The listing builds one solid part. Answer for the finished solid, in the listing's coordinates (mm). Coordinates: 2 decimals unless noted, no trailing zeros. Write each loop counter-clockwise with the first axis right and the second up, starting at its lowest first coordinate (ties: lowest second). Pieces come first, ordered by that corner, then holes. Notation, with made-up numbers: M 25,24 L 55,24 A8 ccw 55,36 Z; hole C -29.75,88 d8. An arc over 180 degrees is marked long. Write item = value, one per line. Start each with the question number.
```python
from build123d import *

# Parameters (mm, degrees)
SKETCH_1_W                 = 28
SKETCH_1_H                 = 8
SKETCH_1_R                 = 1.525
EXTRUDE_1_DEPTH            = 1
SKETCH_3_R                 = 1.525
CUT_EXTRUDE_1_DEPTH        = 10
SKETCH_5_R                 = 1.525
CUT_EXTRUDE_3_DEPTH        = 10
SKETCH_6_R                 = 1.525
CUT_EXTRUDE_4_DEPTH        = 10
EXTRUDE_2_DEPTH            = 1
SKETCH_9_W                 = 55
SKETCH_9_H                 = 4.5
CUT_EXTRUDE_5_DEPTH        = 20.5
FILLET_1_R                 = 2
SKETCH_10_R                = 1.525
CUT_EXTRUDE_6_DEPTH        = 10
SKETCH_11_W                = 28
SKETCH_11_H                = 8
SKETCH_11_R                = 1.525
EXTRUDE_3_DEPTH            = 1
FILLET_2_R                 = 2
SKETCH_12_W                = 29
SKETCH_12_H                = 8
CUT_EXTRUDE_7_DEPTH        = 10
PATTERN_LINEAR_1_OUTLINE_R = 1.525
PATTERN_LINEAR_1_DEPTH     = 1
CUT_EXTRUDE_8_DEPTH        = 10
FILLET_3_R                 = 2
FILLET_4_R                 = 2


with BuildPart() as part:
    # 草图1 → 凸台-拉伸1 (new body)
    # profile 1 of 2: a face of its own
    with BuildSketch(Plane.XY):
        Polygon((-4, 4), (24, 4), (100, 4), (100, 98), (-51, 98), (-51, 4), align=None)
    # profile 2 of 2: a face of its own
    with BuildSketch(Plane.XY):
        with Locations((10, 0)):
            Rectangle(SKETCH_1_W, SKETCH_1_H)
        with Locations((20, 0)):
            Circle(SKETCH_1_R, mode=Mode.SUBTRACT)
        Circle(SKETCH_1_R, mode=Mode.SUBTRACT)
    extrude(amount=EXTRUDE_1_DEPTH)

    # 草图3 → 切除-拉伸1 (cut)
    with BuildSketch(Plane.XY.offset(1)):
        with Locations((-48, 76.75)):
            Circle(SKETCH_3_R)
        with Locations((-48, 56.75)):
            Circle(SKETCH_3_R)
    extrude(amount=-CUT_EXTRUDE_1_DEPTH, mode=Mode.SUBTRACT)

    # 草图5 → 切除-拉伸3 (cut)
    with BuildSketch(Plane.XY.offset(1)):
        with Locations((-41, 95)):
            Circle(SKETCH_5_R)
        with Locations((-21, 95)):
            Circle(SKETCH_5_R)
    extrude(amount=-CUT_EXTRUDE_3_DEPTH, mode=Mode.SUBTRACT)

    # 草图6 → 切除-拉伸4 (cut)
    with BuildSketch(Plane.XY.offset(1)):
        with Locations((41, 95)):
            Circle(SKETCH_6_R)
        with Locations((61, 95)):
            Circle(SKETCH_6_R)
    extrude(amount=-CUT_EXTRUDE_4_DEPTH, mode=Mode.SUBTRACT)

    # 草图7 → 凸台-拉伸2 (add)
    with BuildSketch(Plane.XY.offset(1)):
        Polygon((100, 98), (125.187224089, 4), (100, 4), align=None)
    extrude(amount=-EXTRUDE_2_DEPTH)

    # 草图9 → 切除-拉伸5 (cut)
    with BuildSketch(Plane.XY.offset(1)):
        with Locations((97.687224089, 6.25)):
            Rectangle(SKETCH_9_W, SKETCH_9_H)
    extrude(amount=-CUT_EXTRUDE_5_DEPTH, mode=Mode.SUBTRACT)

    # 圆角1
    fillet_1_edges = [part.edges().sort_by_distance(p)[0] for p in [
        (24, 4, 0.5),
        (24, -4, 0.5),
        (-4, -4, 0.5),
        (-4, 4, 0.5),
        (-51, 4, 0.5),
        (-51, 98, 0.5),
        (100, 98, 0.5),
        (123.981452723, 8.5, 0.5),
        (70.187224089, 4, 0.5),
        (70.187224089, 8.5, 0.5),
    ]]
    fillet(fillet_1_edges, radius=FILLET_1_R)

    # 草图10 → 切除-拉伸6 (cut)
    with BuildSketch(Plane.XY.offset(1)):
        with Locations((60, 34.5)):
            Circle(SKETCH_10_R)
        with Locations((60, 54.5)):
            Circle(SKETCH_10_R)
    extrude(amount=-CUT_EXTRUDE_6_DEPTH, mode=Mode.SUBTRACT)

    # 草图11 → 凸台-拉伸3 (add)
    with BuildSketch(Plane.XY.offset(1)):
        with Locations((-17, 0)):
            Rectangle(SKETCH_11_W, SKETCH_11_H)
        with Locations((-27, 0)):
            Circle(SKETCH_11_R, mode=Mode.SUBTRACT)
        with Locations((-7, 0)):
            Circle(SKETCH_11_R, mode=Mode.SUBTRACT)
    extrude(amount=-EXTRUDE_3_DEPTH)

    # 圆角2
    # the kernel refuses this fillet: 2 mm, written as the material it adds along each edge
    with BuildSketch(Plane(origin=(-31, 4, 1), x_dir=(-1, 0, 0), z_dir=(0, 0, -1))) as fillet_2_piece_1:
        with BuildLine():
            CenterArc((FILLET_2_R, -FILLET_2_R), FILLET_2_R, 90, 90)
            Line((0, -FILLET_2_R), (0, 0))
            Line((0, 0), (FILLET_2_R, 0))
        make_face()
    extrude(amount=1)
    # the kernel refuses this fillet: 2 mm, written as the material it takes off along each edge
    with BuildSketch(Plane(origin=(-3, -4, 3.5), x_dir=(-1, 0, 0), z_dir=(0, 0, -1))) as fillet_2_2_piece_1:
        with BuildLine():
            CenterArc((1, 2), FILLET_2_R, 240, 30)
            Line((0, 0.267949192), (0, 0))
            Line((0, 0), (1, 0))
        make_face()
    extrude(amount=6, mode=Mode.SUBTRACT)
    with BuildSketch(Plane(origin=(-31, -4, 6), x_dir=(0, 1, 0), z_dir=(0, 0, -1))) as fillet_2_2_piece_2:
        with BuildLine():
            CenterArc((FILLET_2_R, FILLET_2_R), FILLET_2_R, 180, 90)
            Line((0, FILLET_2_R), (0, 0))
            Line((0, 0), (FILLET_2_R, 0))
        make_face()
    extrude(amount=11, mode=Mode.SUBTRACT)

    # 草图12 → 切除-拉伸7 (cut)
    with BuildSketch(Plane.XY.offset(1)):
        with Locations((11.5, 0)):
            Rectangle(SKETCH_12_W, SKETCH_12_H)
    extrude(amount=-CUT_EXTRUDE_7_DEPTH, mode=Mode.SUBTRACT)

    # 阵列(线性)1: read off the stored shape, not the designer's step
    # 阵列(线性)1 outline → 阵列(线性)1 (add)
    with BuildSketch(Plane.XY):
        with BuildLine():
            ThreePointArc((24, -2), (24.585786438, -3.414213562), (26, -4))
            Line((26, -4), (50, -4))
            ThreePointArc((50, -4), (51.414213562, -3.414213562), (52, -2))
            Line((52, -2), (52, 4))
            Line((52, 4), (22, 4))
            ThreePointArc((22, 4), (23.414213562, 3.414213562), (24, 2))
            Line((24, 2), (24, -2))
        make_face()
        with Locations((28, 0)):
            Circle(PATTERN_LINEAR_1_OUTLINE_R, mode=Mode.SUBTRACT)
        with Locations((48, 0)):
            Circle(PATTERN_LINEAR_1_OUTLINE_R, mode=Mode.SUBTRACT)
    extrude(amount=PATTERN_LINEAR_1_DEPTH)

    # 草图13 → 切除-拉伸8 (cut)
    with BuildSketch(Plane.XY.offset(1)):
        with BuildLine():
            ThreePointArc((-3, 0), (-4.171572875, -2.828427125), (-7, -4))
            Line((-7, -4), (-4, -4))
            ThreePointArc((-4, -4), (-3.48236191, -3.931851653), (-3, -3.732050808))
            Line((-3, -3.732050808), (-3, 0))
        make_face()
    extrude(amount=-CUT_EXTRUDE_8_DEPTH, mode=Mode.SUBTRACT)

    # 圆角3
    fillet_3_edges = [part.edges().sort_by_distance(p)[0] for p in [
        (-3, 4, 0.5),
    ]]
    fillet(fillet_3_edges, radius=FILLET_3_R)

    # 圆角4
    fillet_4_edges = [part.edges().sort_by_distance(p)[0] for p in [
        (52, 4, 0.5),
    ]]
    fillet(fillet_4_edges, radius=FILLET_4_R)


solid = part.part
```
1. Each of these flat-tipped pins is pushed along its axis until it touches: pin 1 (1.8 mm diameter, centred on x = 60, y = 54.5, fed in from -Z); pin 2 (0.6 mm diameter, centred on y = 6.5, z = 0.5, fed in from +X); pin 3 (0.5 mm diameter, centred on x = 57.5, z = 0.5, fed in from -Y). Where does it stop, or does it pass through?
2. The part is cut by section C-C, the plane y = 46. Write down the section's boundary in (x, z).
3. The part is cut by section B-B, the plane x = 85. Write down the section's boundary in (y, z), and give its area (3 significant figures).
4. Straight lines are drawn through the part: L1, parallel to Y at x = 48, z = 0.4 (3 decimals); L2, parallel to Y at x = 88.5, z = 0.25; L3, parallel to Y at x = -21, z = 0.65 (3 decimals). For each, find the intervals that lie inside material, in ascending order. Write a range as [from, to].
5. For a pull along Y with two mould halves and no side action, classify faces 1 (the face through (35, 48, 0)), 2 (the face through (-4.141, -2.797, 0.507)), 3 (the face through (26.476, 0.067, 0.493)) as pulls with the +Y half, pulls with the -Y half, needs draft (parallel to the pull), parting line crosses it, or undercut.
6. The part is cut by section A-A, the plane z = 0.8. Count the separate pieces of the cut face and the enclosed holes in it, and give its area (3 significant figures).
Solution:
q1.pin_1 = through
q1.pin_2 = 70.21
q1.pin_3 = 4
q2.outline = M -51,0 L 113.93,0 L 113.93,1 L -51,1 Z
q3.outline = M 8.5,0 L 98,0 L 98,1 L 8.5,1 Z
q3.area = 89.5 mm^2
q4.L1 = [-4, -1.525], [1.525, 98]
q4.L2 = [8.5, 98]
q4.L3 = [-4, 93.475], [96.525, 98]
q5.face_1 = needs draft
q5.face_2 = pulls with the -Y half
q5.face_3 = undercut
q6.separate_pieces = 1
q6.enclosed_holes = 12
q6.area = 15,500 mm^2
